from build123d import *

# Parameters (mm, degrees)
SKETCH1_W           = 54.72
SKETCH1_H           = 26.686
BOSS_EXTRUDE1_DEPTH = 15
SKETCH2_W           = 5
SKETCH2_H           = 5
CUT_EXTRUDE1_DEPTH  = 55.19428933
SKETCH3_R           = 1.5
CUT_EXTRUDE2_DEPTH  = 25
CUT_EXTRUDE3_DEPTH  = 3
CUT_EXTRUDE5_DEPTH  = 7
FILLET2_R           = 5


with BuildPart() as part:
    # Sketch1 → Boss-Extrude1 (new body)
    with BuildSketch(Plane.XY):
        with Locations((17.36, 8.343)):
            Rectangle(SKETCH1_W, SKETCH1_H)
        Polygon((0, 0), (0, 12), (3.02, 16.686), (5.22, 16.686), (8.24, 12), (8.24, 0), align=None, mode=Mode.SUBTRACT)
        Polygon((18.46, 16.686), (21.48, 12), (21.48, 0), (13.24, 0), (13.24, 12), (16.26, 16.686), align=None, mode=Mode.SUBTRACT)
        Polygon((31.7, 16.686), (34.72, 12), (34.72, 0), (26.48, 0), (26.48, 12), (29.5, 16.686), align=None, mode=Mode.SUBTRACT)
    extrude(amount=BOSS_EXTRUDE1_DEPTH)

    # Sketch2 → Cut-Extrude1 (cut, through all)
    with BuildSketch(Plane(origin=(0, -5, 0), x_dir=(-1, 0, 0), z_dir=(0, -1, 0))):
        with Locations((7.5, -12.5)):
            Rectangle(SKETCH2_W, SKETCH2_H)
        with Locations((-42.22, -12.5)):
            Rectangle(SKETCH2_W, SKETCH2_H)
    extrude(amount=-CUT_EXTRUDE1_DEPTH, mode=Mode.SUBTRACT)

    # Sketch3 → Cut-Extrude2 (cut)
    with BuildSketch(Plane.XY.offset(10)):
        with Locations((-7.5, 7.331502285)):
            Circle(SKETCH3_R)
        with Locations((42.22, 7.331502285)):
            Circle(SKETCH3_R)
    extrude(amount=-CUT_EXTRUDE2_DEPTH, mode=Mode.SUBTRACT)

    # Sketch4 → Cut-Extrude3 (cut)
    with BuildSketch(Plane.XY.offset(10)):
        Polygon((-7.5, 10.651266332), (-10.375, 8.991384309), (-10.375, 5.671620261), (-7.5, 4.011738237), (-4.625, 5.671620261), (-4.625, 8.991384309), align=None)
        Polygon((42.22, 10.651266332), (39.345, 8.991384309), (39.345, 5.671620261), (42.22, 4.011738237), (45.095, 5.671620261), (45.095, 8.991384309), align=None)
    extrude(amount=-CUT_EXTRUDE3_DEPTH, mode=Mode.SUBTRACT)

    # Sketch7 → Cut-Extrude5 (cut)
    with BuildSketch(Plane(origin=(0, 0, 0), x_dir=(-1, 0, 0), z_dir=(0, 0, -1))):
        Polygon((0, 0), (-7.36, 0), (-7.36, -5), (-27.36, -5), (-27.36, 0), (-34.72, 0), (-34.72, 16.686), (0, 16.686), align=None)
    extrude(amount=-CUT_EXTRUDE5_DEPTH, mode=Mode.SUBTRACT)

    # Fillet2
    # the kernel refuses this fillet: 5 mm, written as the material it adds along each edge
    with BuildSketch(Plane(origin=(-5, -5, 10), x_dir=(-1, 0, 0), z_dir=(0, 1, 0))) as fillet2_piece_1_section:
        with BuildLine():
            CenterArc((FILLET2_R, FILLET2_R), FILLET2_R, 180, 90)
            Line((0, FILLET2_R), (0, 0))
            Line((0, 0), (FILLET2_R, 0))
        make_face()
    fillet2_piece_1 = extrude(amount=22.95511391, mode=Mode.PRIVATE)
    fillet2_piece_1 = split(fillet2_piece_1, bisect_by=Plane(origin=(-4.358665605, 2.198087978, 11.088883398), z_dir=(-0.5, -0.8660254037844387, 0)), keep=Keep.TOP, mode=Mode.PRIVATE)
    add(fillet2_piece_1)
    with BuildSketch(Plane(origin=(-5, -17.5, 10), x_dir=(-1, 0, 0), z_dir=(0, 1, 0))) as fillet2_piece_2_section:
        with BuildLine():
            CenterArc((FILLET2_R, FILLET2_R), FILLET2_R, 180, 90)
            Line((0, FILLET2_R), (0, 0))
            Line((0, 0), (FILLET2_R, 0))
        make_face()
    fillet2_piece_2 = extrude(amount=35.45511391, mode=Mode.PRIVATE)
    fillet2_piece_2 = split(fillet2_piece_2, bisect_by=Plane(origin=(-6.083354929, 4.82963865, 11.432065422), z_dir=(0.49999999999999967, -0.8660254037844388, 0)), keep=Keep.TOP, mode=Mode.PRIVATE)
    fillet2_piece_2 = split(fillet2_piece_2, bisect_by=Plane(origin=(-6.083354929, 3.193837824, 11.432065422), z_dir=(0.5, 0.8660254037844387, 0)), keep=Keep.TOP, mode=Mode.PRIVATE)
    add(fillet2_piece_2)
    with BuildSketch(Plane(origin=(-5, -17.5, 10), x_dir=(-1, 0, 0), z_dir=(0, 1, 0))) as fillet2_piece_3_section:
        with BuildLine():
            CenterArc((FILLET2_R, FILLET2_R), FILLET2_R, 180, 90)
            Line((0, FILLET2_R), (0, 0))
            Line((0, 0), (FILLET2_R, 0))
        make_face()
    fillet2_piece_3 = extrude(amount=35.45511391, mode=Mode.PRIVATE)
    fillet2_piece_3 = split(fillet2_piece_3, bisect_by=Plane(origin=(-6.083354929, 9.83336592, 11.432065422), z_dir=(0.5000000000000001, 0.8660254037844387, 0)), keep=Keep.TOP, mode=Mode.PRIVATE)
    add(fillet2_piece_3)
    with BuildSketch(Plane(origin=(-5, -17.5, 10), x_dir=(-1, 0, 0), z_dir=(0, 1, 0))) as fillet2_piece_4_section:
        with BuildLine():
            CenterArc((FILLET2_R, FILLET2_R), FILLET2_R, 180, 90)
            Line((0, FILLET2_R), (0, 0))
            Line((0, 0), (FILLET2_R, 0))
        make_face()
    fillet2_piece_4 = extrude(amount=35.45511391, mode=Mode.PRIVATE)
    fillet2_piece_4 = split(fillet2_piece_4, bisect_by=Plane(origin=(-8.244164443, 10.221622791, 10.130784203), z_dir=(-0.5000000000000001, 0.8660254037844387, 0)), keep=Keep.TOP, mode=Mode.PRIVATE)
    add(fillet2_piece_4)
    with BuildSketch(Plane(origin=(-5, -3.292109341, 10), x_dir=(-1, 0, 0), z_dir=(0, 1, 0))) as fillet2_piece_5_section:
        with BuildLine():
            CenterArc((FILLET2_R, FILLET2_R), FILLET2_R, 180, 90)
            Line((0, FILLET2_R), (0, 0))
            Line((0, 0), (FILLET2_R, 0))
        make_face()
    fillet2_piece_5 = extrude(amount=37.478109341, mode=Mode.PRIVATE)
    fillet2_piece_5 = split(fillet2_piece_5, bisect_by=Plane(origin=(-8.244164443, 4.441381778, 10.130784203), z_dir=(-0.5, -0.8660254037844387, 0)), keep=Keep.TOP, mode=Mode.PRIVATE)
    add(fillet2_piece_5)
    with BuildSketch(Plane(origin=(-5, -3.292109341, 10), x_dir=(-1, 0, 0), z_dir=(0, 1, 0))) as fillet2_piece_6_section:
        with BuildLine():
            CenterArc((FILLET2_R, FILLET2_R), FILLET2_R, 180, 90)
            Line((0, FILLET2_R), (0, 0))
            Line((0, 0), (FILLET2_R, 0))
        make_face()
    fillet2_piece_6 = extrude(amount=37.478109341, mode=Mode.PRIVATE)
    fillet2_piece_6 = split(fillet2_piece_6, bisect_by=Plane(origin=(-6.083354929, 4.82963865, 11.432065422), z_dir=(0.49999999999999967, -0.8660254037844388, 0)), keep=Keep.TOP, mode=Mode.PRIVATE)
    add(fillet2_piece_6)
    with BuildSketch(Plane(origin=(-5, -3.292109341, 10), x_dir=(-1, 0, 0), z_dir=(0, 1, 0))) as fillet2_piece_7_section:
        with BuildLine():
            CenterArc((FILLET2_R, FILLET2_R), FILLET2_R, 180, 90)
            Line((0, FILLET2_R), (0, 0))
            Line((0, 0), (FILLET2_R, 0))
        make_face()
    fillet2_piece_7 = extrude(amount=24.978109341, mode=Mode.PRIVATE)
    fillet2_piece_7 = split(fillet2_piece_7, bisect_by=Plane(origin=(-6.083354929, 9.83336592, 11.432065422), z_dir=(0.5000000000000001, 0.8660254037844387, 0)), keep=Keep.TOP, mode=Mode.PRIVATE)
    add(fillet2_piece_7)
    with BuildSketch(Plane(origin=(-5, -3.292109341, 10), x_dir=(-1, 0, 0), z_dir=(0, 1, 0))) as fillet2_piece_8_section:
        with BuildLine():
            CenterArc((FILLET2_R, FILLET2_R), FILLET2_R, 180, 90)
            Line((0, FILLET2_R), (0, 0))
            Line((0, 0), (FILLET2_R, 0))
        make_face()
    fillet2_piece_8 = extrude(amount=37.478109341, mode=Mode.PRIVATE)
    fillet2_piece_8 = split(fillet2_piece_8, bisect_by=Plane(origin=(-8.244164443, 11.080909874, 10.130784203), z_dir=(-0.5000000000000001, -0.8660254037844387, 0)), keep=Keep.TOP, mode=Mode.PRIVATE)
    fillet2_piece_8 = split(fillet2_piece_8, bisect_by=Plane(origin=(-8.244164443, 10.221622791, 10.130784203), z_dir=(-0.5000000000000001, 0.8660254037844387, 0)), keep=Keep.TOP, mode=Mode.PRIVATE)
    add(fillet2_piece_8)
    with BuildSketch(Plane(origin=(39.72, -3.292109341, 10), x_dir=(1, 0, 0), z_dir=(0, 1, 0))) as fillet2_piece_9_section:
        with BuildLine():
            CenterArc((FILLET2_R, -FILLET2_R), FILLET2_R, 90, 90)
            Line((0, -FILLET2_R), (0, 0))
            Line((0, 0), (FILLET2_R, 0))
        make_face()
    fillet2_piece_9 = extrude(amount=37.478109341, mode=Mode.PRIVATE)
    fillet2_piece_9 = split(fillet2_piece_9, bisect_by=Plane(origin=(42.964164443, 4.441381778, 10.130784203), z_dir=(0.4999999999999993, -0.866025403784439, 0)), keep=Keep.TOP, mode=Mode.PRIVATE)
    add(fillet2_piece_9)
    with BuildSketch(Plane(origin=(39.72, -3.292109341, 10), x_dir=(1, 0, 0), z_dir=(0, 1, 0))) as fillet2_piece_10_section:
        with BuildLine():
            CenterArc((FILLET2_R, -FILLET2_R), FILLET2_R, 90, 90)
            Line((0, -FILLET2_R), (0, 0))
            Line((0, 0), (FILLET2_R, 0))
        make_face()
    fillet2_piece_10 = extrude(amount=37.478109341, mode=Mode.PRIVATE)
    fillet2_piece_10 = split(fillet2_piece_10, bisect_by=Plane(origin=(40.803354929, 4.82963865, 11.432065422), z_dir=(-0.5000000000000001, -0.8660254037844386, 0)), keep=Keep.TOP, mode=Mode.PRIVATE)
    add(fillet2_piece_10)
    with BuildSketch(Plane(origin=(39.72, -3.292109341, 10), x_dir=(1, 0, 0), z_dir=(0, 1, 0))) as fillet2_piece_11_section:
        with BuildLine():
            CenterArc((FILLET2_R, -FILLET2_R), FILLET2_R, 90, 90)
            Line((0, -FILLET2_R), (0, 0))
            Line((0, 0), (FILLET2_R, 0))
        make_face()
    fillet2_piece_11 = extrude(amount=24.978109341, mode=Mode.PRIVATE)
    fillet2_piece_11 = split(fillet2_piece_11, bisect_by=Plane(origin=(40.803354929, 9.83336592, 11.432065422), z_dir=(-0.5, 0.8660254037844387, 0)), keep=Keep.TOP, mode=Mode.PRIVATE)
    add(fillet2_piece_11)
    with BuildSketch(Plane(origin=(39.72, -3.292109341, 10), x_dir=(1, 0, 0), z_dir=(0, 1, 0))) as fillet2_piece_12_section:
        with BuildLine():
            CenterArc((FILLET2_R, -FILLET2_R), FILLET2_R, 90, 90)
            Line((0, -FILLET2_R), (0, 0))
            Line((0, 0), (FILLET2_R, 0))
        make_face()
    fillet2_piece_12 = extrude(amount=37.478109341, mode=Mode.PRIVATE)
    fillet2_piece_12 = split(fillet2_piece_12, bisect_by=Plane(origin=(42.964164443, 11.080909874, 10.130784203), z_dir=(0.5, -0.8660254037844387, 0)), keep=Keep.TOP, mode=Mode.PRIVATE)
    fillet2_piece_12 = split(fillet2_piece_12, bisect_by=Plane(origin=(42.964164443, 10.221622791, 10.130784203), z_dir=(0.4999999999999985, 0.8660254037844396, 0)), keep=Keep.TOP, mode=Mode.PRIVATE)
    add(fillet2_piece_12)
    with BuildSketch(Plane(origin=(39.72, -5, 10), x_dir=(0, 0, 1), z_dir=(0, 1, 0))) as fillet2_piece_13_section:
        with BuildLine():
            CenterArc((FILLET2_R, FILLET2_R), FILLET2_R, 180, 90)
            Line((0, FILLET2_R), (0, 0))
            Line((0, 0), (FILLET2_R, 0))
        make_face()
    fillet2_piece_13 = extrude(amount=22.95511391, mode=Mode.PRIVATE)
    fillet2_piece_13 = split(fillet2_piece_13, bisect_by=Plane(origin=(39.078665605, 2.198087978, 11.088883398), z_dir=(0.4999999999999993, -0.866025403784439, 0)), keep=Keep.TOP, mode=Mode.PRIVATE)
    add(fillet2_piece_13)
    with BuildSketch(Plane(origin=(39.72, -17.5, 10), x_dir=(0, 0, 1), z_dir=(0, 1, 0))) as fillet2_piece_14_section:
        with BuildLine():
            CenterArc((FILLET2_R, FILLET2_R), FILLET2_R, 180, 90)
            Line((0, FILLET2_R), (0, 0))
            Line((0, 0), (FILLET2_R, 0))
        make_face()
    fillet2_piece_14 = extrude(amount=35.45511391, mode=Mode.PRIVATE)
    fillet2_piece_14 = split(fillet2_piece_14, bisect_by=Plane(origin=(40.803354929, 4.82963865, 11.432065422), z_dir=(-0.5000000000000001, -0.8660254037844386, 0)), keep=Keep.TOP, mode=Mode.PRIVATE)
    fillet2_piece_14 = split(fillet2_piece_14, bisect_by=Plane(origin=(40.803354929, 3.193837824, 11.432065422), z_dir=(-0.4999999999999993, 0.866025403784439, 0)), keep=Keep.TOP, mode=Mode.PRIVATE)
    add(fillet2_piece_14)
    with BuildSketch(Plane(origin=(39.72, -17.5, 10), x_dir=(0, 0, 1), z_dir=(0, 1, 0))) as fillet2_piece_15_section:
        with BuildLine():
            CenterArc((FILLET2_R, FILLET2_R), FILLET2_R, 180, 90)
            Line((0, FILLET2_R), (0, 0))
            Line((0, 0), (FILLET2_R, 0))
        make_face()
    fillet2_piece_15 = extrude(amount=35.45511391, mode=Mode.PRIVATE)
    fillet2_piece_15 = split(fillet2_piece_15, bisect_by=Plane(origin=(42.964164443, 10.221622791, 10.130784203), z_dir=(0.4999999999999985, 0.8660254037844396, 0)), keep=Keep.TOP, mode=Mode.PRIVATE)
    add(fillet2_piece_15)
    with BuildSketch(Plane(origin=(39.72, -17.5, 10), x_dir=(0, 0, 1), z_dir=(0, 1, 0))) as fillet2_piece_16_section:
        with BuildLine():
            CenterArc((FILLET2_R, FILLET2_R), FILLET2_R, 180, 90)
            Line((0, FILLET2_R), (0, 0))
            Line((0, 0), (FILLET2_R, 0))
        make_face()
    fillet2_piece_16 = extrude(amount=35.45511391, mode=Mode.PRIVATE)
    fillet2_piece_16 = split(fillet2_piece_16, bisect_by=Plane(origin=(40.803354929, 9.833365919, 11.432065422), z_dir=(-0.5, 0.8660254037844387, 0)), keep=Keep.TOP, mode=Mode.PRIVATE)
    add(fillet2_piece_16)


solid = part.part
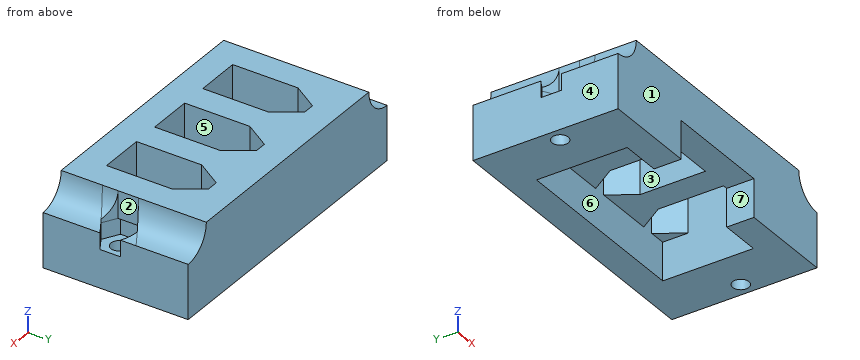
Source: CAD feature listing. Evaluate the final solid. Frame: model axes, mm. Face numbers are marked on the shaded views. A direction names the side the tool comes from. Round coordinates to 2 decimals unless told otherwise and drop trailing zeros. Loops run counter-clockwise (first coordinate to the right, second up) from the corner with the lowest first, then second, coordinate; pieces in that order, holes last. Notation, with made-up numbers: (78.5, -35) -> (93.5, -35) arc R13 cw to (93.5, -20) -> close; hole circle Ø4 at (-29, -24.5). An arc over 180 degrees is marked (long way). Answer as a JSON object with one key per item and string values. Group by question number.
Q1. Mould query, pull axis X, two halves, no side actions, for the marked faces 1, 2, 3 and 4. Classes: pulls with the +X half, pulls with the -X half, needs draft (parallel to the pull), parting line crosses it, or undercut.
Q2. Access query for the marked faces 5, 6 and 7. Directions: +Z, -Z, +X, -X, +Y, -Y. A direction counts if a zero-diameter tool reaches every point of the face in a straight line with its end or side. Return the directions, or none.
Q3. Section query C-C (z = 14). State how many separate pieces and enclosed holes the cut face has, plus the area to 3 significant figures.
Q4. Section query B-B (y = -1). Output: boundary loops of the cut face in (x, z), plus the area to 3 significant figures.
Q5. Ray query, line 1 (X direction, y = 10.75, z = 12); line 2 (Y direction, x = 1, z = 3.5); line 3 (Y direction, x = -7.5, z = 3.75). Return the intervals inside material, ascending. Write a range as from..to.
Q6. Contact query for flat-ended pins moving along their axis: P1, Ø0.9, axis at y = 7, z = 8, coming from the +X side (3 decimals); P2, Ø4, axis at y = 7.5, z = 13.5, coming from the -X side; P3, Ø3, axis at y = 7.5, z = 13.5, coming from the +X side. Output: stop coordinate, or through.
Q7. Section query D-D (z = 3.75). Output: boundary loops of the cut face in (x, y).
Q8. Section query A-A (x = 15). Output: boundary loops of the cut face in (y, z), plus the area to 3 significant figures.
Completed:
{
 "1": {"face 1": "needs draft", "face 2": "pulls with the +X half", "face 3": "undercut", "face 4": "pulls with the -X half"},
 "2": {"face 5": "+Z, -Z", "face 6": "-Z", "face 7": "-Z, -Y"},
 "3": {"separate pieces": "1", "enclosed holes": "3", "area": "828 mm²"},
 "4": {"outline": "(-10, 0) -> (7.36, 0) -> (7.36, 7) -> (27.36, 7) -> (27.36, 0) -> (44.72, 0) -> (44.72, 10) arc R5 cw to (39.72, 15) -> (-5, 15) arc R5 cw to (-10, 10) -> close", "area": "642 mm²"},
 "5": {"line 1": "-6..0, 8.24..13.24, 21.48..26.48, 34.72..40.72", "line 2": "-5..0, 16.69..21.69", "line 3": "-5..5.83, 8.83..21.69"},
 "6": {"P1": "x = 39.345", "P2": "x = -5.41", "P3": "x = 39.72"},
 "7": {"outline": "(-10, -5) -> (7.36, -5) -> (7.36, 0) -> (0, 0) -> (0, 16.69) -> (34.72, 16.69) -> (34.72, 0) -> (27.36, 0) -> (27.36, -5) -> (44.72, -5) -> (44.72, 21.69) -> (-10, 21.69) -> close; hole circle Ø3 at (-7.5, 7.33); hole circle Ø3 at (42.22, 7.33)"},
 "8": {"outline": "(-5, 7) -> (0, 7) -> (0, 15) -> (-5, 15) -> close; (14.73, 7) -> (16.69, 7) -> (16.69, 0) -> (21.69, 0) -> (21.69, 15) -> (14.73, 15) -> close", "area": "131 mm²"}
}
